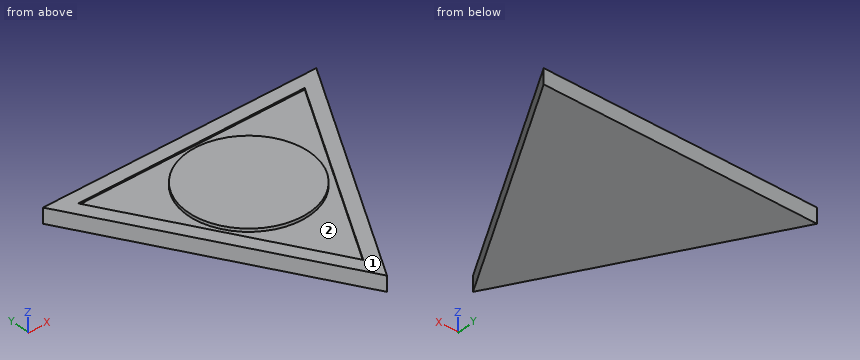
from build123d import *

# Parameters (mm, degrees)
F2_DEPTH = 5
F0_R     = 20.5
F3_DEPTH = 5
F4_T     = -4.5
F5_R     = 20
F6_DEPTH = 1


with BuildPart() as f2:
    # F1 (on Top) → F2 (new body)
    with BuildSketch(Plane.XY):
        Polygon((45.466336, 26.250001), (-45.466336, 26.250001), (0, -52.500002), align=None)
    extrude(amount=F2_DEPTH)

    # F0 (on Top) → F3 (join)
    with BuildSketch(Plane.XY):
        Circle(F0_R)
    extrude(amount=F3_DEPTH)

    # F4
    f4_openings = [f2.faces().sort_by_distance(p)[0] for p in [
        (0, 0, 5),
    ]]
    offset(amount=F4_T, openings=f4_openings)

    # F5 (on face) → F6 (join)
    with BuildSketch(Plane.XY.offset(4.5)):
        Circle(F5_R)
    extrude(amount=F6_DEPTH)


solid = f2.part
Can you work these out from the model? Positions are in its coordinate system, mm. Face numbers are marked on the shaded views. Coordinates: 2 decimals unless noted, no trailing zeros. Write each loop counter-clockwise with the first axis right and the second up, starting at its lowest first coordinate (ties: lowest second). Pieces come first, ordered by that corner, then holes. Notation, with made-up numbers: (78.25, 5.5) - (109.25, 5.5) arc R14 cw to (109.25, 22.5) - close; hole circle Ø10 at (18.25, -34). An arc over 180 degrees is marked (long way). Return JSON: item names as keys, results as strings. Group by question number.
Item 1: Please list where these lines run through material, in increasing order: probe 1 along Z at (x, y) = (17, -15); probe 2 along X at (y, z) = (-31.5, 4.9); probe 3 along Y at (x, z) = (-21.5, 4.8).
Item 2: I'm going to push flat-ended pins straight in: pin 1 Ø1.5 at (y, z) = (12, 0.5) entering from -X; pin 2 Ø1 at (y, z) = (-3, 2.5) entering from -X; pin 3 Ø1 at (x, y) = (-16, 16.5) entering from +Z. Where does each tip first touch, or does it pass through?
Item 3: If we section it at C-C (z = 1.9): Write out the boundary of the cut face in (x, y).
Item 4: If we section it at B-B (x = -10.5): Write out the boundary of the cut face in (y, z), then the cut area to 3 significant figures.
Item 5: If we section it at D-D (y = 0): Write out the boundary of the cut face in (x, z).
Item 6: If we section it at A-A (y = -33): Write out the boundary of the cut face in (x, z).
Item 7: We'd pull the mould along X, two halves only. Please class the marked faces 1 and 2: pulls with the +X half, pulls with the -X half, needs draft (parallel to the pull), parting line crosses it, or undercut.
Return value:
{
 "1": {"probe 1": "z = 0 to 5", "probe 2": "x = -12.12 to -6.93, 6.93 to 12.12", "probe 3": "y = -15.26 to -6.26, 21.75 to 26.25"},
 "2": {"pin 1": "stops at x = -37.67", "pin 2": "stops at x = -28.87", "pin 3": "stops at z = 4.5"},
 "3": {"outline": "(-45.47, 26.25) - (0, -52.5) - (45.47, 26.25) - close"},
 "4": {"outline": "(-34.31, 0) - (26.25, 0) - (26.25, 5) - (21.75, 5) - (21.75, 4.5) - (17.02, 4.5) - (17.02, 5.5) - (-17.02, 5.5) - (-17.02, 4.5) - (-25.31, 4.5) - (-25.31, 5) - (-34.31, 5) - close", "area": "313 mm^2"},
 "5": {"outline": "(-30.31, 0) - (30.31, 0) - (30.31, 5) - (25.11, 5) - (25.11, 4.5) - (20, 4.5) - (20, 5.5) - (-20, 5.5) - (-20, 4.5) - (-25.11, 4.5) - (-25.11, 5) - (-30.31, 5) - close"},
 "6": {"outline": "(-11.26, 0) - (11.26, 0) - (11.26, 5) - (6.06, 5) - (6.06, 4.5) - (-6.06, 4.5) - (-6.06, 5) - (-11.26, 5) - close"},
 "7": {"face 1": "needs draft", "face 2": "undercut"}
}
